Design review of the part built by this model. Coordinates are the model's own, in mm. A direction names the side the tool comes from. Give positions to 0.01 mm unless a question says otherwise; leave off trailing zeros. Loops run counter-clockwise (first coordinate to the right, second up) from the corner with the lowest first, then second, coordinate; pieces in that order, holes last. Notation, with made-up numbers: (54.5, 82) - (70.5, 82) arc R16 cw to (70.5, 105) - close; hole circle Ø11 at (-31.75, 36). An arc over 180 degrees is marked (long way). Write each question's results on one line, items separated by ' | '.
from build123d import *

# Parameters (mm, degrees)
F1_DEPTH = 3.4163
F3_DEPTH = 457.2
F4_R     = 50.8
F5_DEPTH = 25.4


with BuildPart() as f1:
    # F0 (on Front) → F1 (new body)
    with BuildSketch(Plane.XZ):
        Polygon((0, 457.2), (0, 0), (304.8, 0), align=None)
    extrude(amount=F1_DEPTH)

    # F2 (on Top) → F3 (join, through all)
    with BuildSketch(Plane.XY):
        Polygon((0, -3.4163), (0, 0), (-38.1, 0), (-38.1, 41.0337), (-41.5163, 41.0337), (-41.5163, -3.4163), align=None)
    extrude(amount=F3_DEPTH)

    # F4 (on face) → F5 (cut)
    with BuildSketch(Plane.XZ.offset(3.4163)):
        with Locations((136.2837, 0)):
            Circle(F4_R)
    extrude(amount=-F5_DEPTH, mode=Mode.SUBTRACT)


solid = f1.part
(1) Wall thickness on line 1 along Y through (x, z) = (-7, 135); line 2 along X through (y, z) = (28.5, 20); line 3 along X through (y, z) = (-2, 254): over which ranges is each line inside the solid? List them lowest first. Write a range as from..to.
Answers below:
line 1: -3.42..0 | line 2: -41.52..-38.1 | line 3: -41.52..135.47
(2) Insertion check: P1, Ø5, axis at x = 268.5, z = 46, coming from the +Y side; P2, Ø3, axis at y = 24.5, z = 381.5, coming from the +X side. Each pin has a flat end and moves straight along its axis. Give the tip position at first contact, or say it passes through.
Answers below:
P1: y = 0 | P2: x = -38.1
(3) Take a section at A-A on z = 132. Give the boundary of the cut face in (x, y).
Answers below:
outline: (-41.52, -3.42) - (216.8, -3.42) - (216.8, 0) - (-38.1, 0) - (-38.1, 41.03) - (-41.52, 41.03) - close
(4) Take a section at D-D on z = 328. Give the boundary of the cut face in (x, y), plus the area to 3 significant figures.
Answers below:
outline: (-41.52, -3.42) - (86.13, -3.42) - (86.13, 0) - (-38.1, 0) - (-38.1, 41.03) - (-41.52, 41.03) - close | area: 576 mm2
(5) Tool access review of faces 1 (the flat face through (3, -1, 0)), 2 (the flat face through (-38.1, 20, 225)): name each direction out of +Z, -Z, +X, -X, +Y, -Y from which nothing blocks a thin tool from reaching the whole face with its end or side.
Answers below:
face 1: -Z, +X, -X, +Y, -Y | face 2: +Z, -Z, +X, +Y
(6) Take a section at B-B on x = 239.5. Give the boundary of the cut face in (y, z).
Answers below:
outline: (-3.42, 0) - (0, 0) - (0, 97.95) - (-3.42, 97.95) - close
(7) Draft analysis for pull direction X (two halves, no side actions). For faces 3 (the cylindrical face through (137.401, -1.732, 50.788)), 4 (the flat face through (91, -3.416, 175)), 5 (the flat face through (-41.516, 19, 225)), state which applies: pulls with the +X half, pulls with the -X half, needs draft (parallel to the pull), parting line crosses it, or undercut.
Answers below:
face 3: undercut | face 4: needs draft | face 5: pulls with the -X half
(8) Take a section at C-C on y = 13. Give the boundary of the cut face in (x, z).
Answers below:
outline: (-41.52, 0) - (-38.1, 0) - (-38.1, 457.2) - (-41.52, 457.2) - close
